from build123d import *

# Parameters (mm, degrees)
STOK_DYS_START             = 4.792312704
STOK_DYS_BE1806_13_1_DEPTH = 8.707687296
IZIM1_R                    = 1.5
KES_EKSTR_ZYON1_DEPTH      = 10


# Read off the part's stored shape, not the designer's step: Stok-DYS BE1806-13-1
with BuildPart() as part:
    # Stok-DYS BE1806-13-1 outline → Stok-DYS BE1806-13-1 (new body)
    with BuildSketch(Plane.XY.offset(STOK_DYS_START)):
        Polygon((2, 7.5), (2, 8), (-2, 8), (-2, 7.5), (-0.5, 7.5), (-0.5, 1.702843619), (-3.634179365, 6.579721905), (-2.372299065, 7.390683131), (-2.642619474, 7.811309898), (-6.007633605, 5.648746628), (-5.737313197, 5.228119861), (-4.475432897, 6.039081088), (-1.341253533, 1.162202802), (-6.614532459, 3.570428595), (-5.991409939, 4.934876588), (-6.446225937, 5.142584095), (-8.107885989, 1.504056113), (-7.653069991, 1.296348607), (-7.029947472, 2.6607966), (-1.756668546, 0.252570807), (-7.494818233, -0.572450566), (-7.708290491, 0.912281597), (-8.203201212, 0.841124178), (-7.633941859, -3.11816159), (-7.139031138, -3.047004171), (-7.352503395, -1.562272008), (-1.614353708, -0.737250635), (-5.995552175, -4.533580717), (-6.977843276, -3.399956356), (-7.355718063, -3.727386723), (-4.736275127, -6.75038502), (-4.35840034, -6.422954653), (-5.340691441, -5.289330292), (-0.959492974, -1.49300021), (-2.592740663, -7.055331024), (-4.031980124, -6.632732188), (-4.172846402, -7.112478675), (-0.334874508, -8.239408903), (-0.194008229, -7.759662416), (-1.63324769, -7.337063581), (0, -1.774732766), (1.63324769, -7.337063581), (0.194008229, -7.759662416), (0.334874508, -8.239408903), (4.172846402, -7.112478675), (4.031980124, -6.632732188), (2.592740663, -7.055331024), (0.959492974, -1.49300021), (5.340691441, -5.289330292), (4.35840034, -6.422954653), (4.736275127, -6.75038502), (7.355718063, -3.727386723), (6.977843276, -3.399956356), (5.995552175, -4.533580717), (1.614353708, -0.737250635), (7.352503395, -1.562272008), (7.139031138, -3.047004171), (7.633941859, -3.11816159), (8.203201212, 0.841124178), (7.708290491, 0.912281597), (7.494818233, -0.572450566), (1.756668546, 0.252570807), (7.029947472, 2.6607966), (7.653069991, 1.296348607), (8.107885989, 1.504056113), (6.446225937, 5.142584095), (5.991409939, 4.934876588), (6.614532459, 3.570428595), (1.341253533, 1.162202802), (4.475432897, 6.039081088), (5.737313197, 5.228119861), (6.007633605, 5.648746628), (2.642619474, 7.811309898), (2.372299065, 7.390683131), (3.634179364, 6.579721905), (0.5, 1.702843619), (0.5, 7.5), align=None)
    extrude(amount=STOK_DYS_BE1806_13_1_DEPTH)

    # Çizim1 → Kes-Ekstrüzyon1 (cut)
    with BuildSketch(Plane.XY.offset(13.5)):
        Circle(IZIM1_R)
    extrude(amount=-KES_EKSTR_ZYON1_DEPTH, mode=Mode.SUBTRACT)


solid = part.part
Geometry check sheet. Reference: the model listing, model coordinates, mm. A direction names the side the tool comes from. Give positions to 0.01 mm unless a question says otherwise; leave off trailing zeros. Loops run counter-clockwise (first coordinate to the right, second up) from the corner with the lowest first, then second, coordinate; pieces in that order, holes last. Notation, with made-up numbers: M -21,20.5 L 11,20.5 A19 cw 11,35.5 Z; hole C 71.25,64 d7. An arc over 180 degrees is marked long. Answer as a JSON object with one key per item and string values. Group by question number.
Item 1: Sectioned sample at D-D on x = 5. Record the boundary of the cut face in (y, z).
Item 2: Mould release check, pull along X, two halves, no side actions. Record for faces 1 (the flat face through (-3.181, -3.418, 9.085)), 2 (the flat face through (-7.923, -1.111, 9.085)), 3 (the flat face through (7.289, 3.298, 9.085)): pulls with the +X half, pulls with the -X half, needs draft (parallel to the pull), parting line crosses it, or undercut.
Item 3: Sectioned sample at A-A on y = -5.5. Record the boundary of the cut face in (x, z).
Item 4: Sectioned sample at C-C on x = -0.75. Record the boundary of the cut face in (y, z).
Item 5: Material ranges on L1, parallel to X at y = -2.75, z = 10.25; L2, parallel to X at y = 6.5, z = 6; L3, parallel to X at y = -6, z = 8.75, recorded low to high.
Item 6: Sectioned sample at B-B on x = -3.25. Record the boundary of the cut face in (y, z).
Item 7: Access from +Z, -Z, +X, -X, +Y, -Y to the whole of each face (thin tool, end or side, straight path). Record for faces 4 (the flat face through (3.32, -6.84, 9.09)), 5 (the flat face through (6.03, -5.26, 9.09)).
Item 8: Gauge pin test, flat ends, axial feed: pin 1 (1 mm diameter, centred on y = -2, z = 10.5, fed in from -X); pin 2 (0.8 mm diameter, centred on x = -1, z = 10.5, fed in from -Y); pin 3 (0.6 mm diameter, centred on y = 7.5, z = 7.5, fed in from +X). Record the tip position at first contact, or that the pin passes through.
Findings below:
{
 "1": {"outline": "M -6.45,4.79 L -5.68,4.79 L -5.68,13.5 L -6.45,13.5 Z; M -4.99,4.79 L -3.67,4.79 L -3.67,13.5 L -4.99,13.5 Z; M -1.22,4.79 L -0.21,4.79 L -0.21,13.5 L -1.22,13.5 Z; M 1.73,4.79 L 2.83,4.79 L 2.83,13.5 L 1.73,13.5 Z; M 5.7,4.79 L 6.3,4.79 L 6.3,13.5 L 5.7,13.5 Z"},
 "2": {"face 1": "undercut", "face 2": "pulls with the -X half", "face 3": "pulls with the +X half"},
 "3": {"outline": "M -5.82,4.79 L -5.16,4.79 L -5.16,13.5 L -5.82,13.5 Z; M -2.14,4.79 L -1.09,4.79 L -1.09,13.5 L -2.14,13.5 Z; M 1.09,4.79 L 2.14,4.79 L 2.14,13.5 L 1.09,13.5 Z; M 5.16,4.79 L 5.82,4.79 L 5.82,13.5 L 5.16,13.5 Z"},
 "4": {"outline": "M -8.12,4.79 L -7.6,4.79 L -7.6,13.5 L -8.12,13.5 Z; M -4.33,4.79 L -1.3,4.79 L -1.3,13.5 L -4.33,13.5 Z; M 1.3,4.79 L 2.09,4.79 L 2.09,13.5 L 1.3,13.5 Z; M 7.5,4.79 L 8,4.79 L 8,13.5 L 7.5,13.5 Z"},
 "5": {"L1": "-7.69 to -7.18, -3.94 to -2.41, -1.33 to -0.29, 0.29 to 1.33, 2.41 to 3.94, 7.18 to 7.69", "L2": "-4.68 to -3.58, -0.5 to 0.5, 3.58 to 4.68", "L3": "-5.39 to -4.72, -2.28 to -1.24, 1.24 to 2.28, 4.72 to 5.39"},
 "6": {"outline": "M -7.38,4.79 L -6.86,4.79 L -6.86,13.5 L -7.38,13.5 Z; M -3.48,4.79 L -2.15,4.79 L -2.15,13.5 L -3.48,13.5 Z; M -0.97,4.79 L 0.04,4.79 L 0.04,13.5 L -0.97,13.5 Z; M 0.93,4.79 L 2.03,4.79 L 2.03,13.5 L 0.93,13.5 Z; M 4.13,4.79 L 5.98,4.79 L 5.98,13.5 L 4.13,13.5 Z; M 6.83,4.79 L 7.42,4.79 L 7.42,13.5 L 6.83,13.5 Z"},
 "7": {"face 4": "+Z, -Z", "face 5": "+Z, -Z, +X, -Y"},
 "8": {"pin 1": "x = -7.87", "pin 2": "y = -8.16", "pin 3": "x = 3.59"}
}
